Check sheet for the modelled part. Datum: model origin and axes. Units: mm. A direction names the side the tool comes from. Round coordinates to 2 decimals unless told otherwise and drop trailing zeros. Loops run counter-clockwise (first coordinate to the right, second up) from the corner with the lowest first, then second, coordinate; pieces in that order, holes last. Notation, with made-up numbers: (30, 9) - (42, 9) arc R10 ccw to (42, 22) - close; hole circle Ø10 at (49.25, -6.5). An arc over 180 degrees is marked (long way). Put each result on its own line as item: value. Start each with the question number.
Item 1: Tool access check on faces 4 (the flat face through (-7, 0, 0)), 5 (the flat face through (-6.096, 13, 0)). Record the directions out of +Z, -Z, +X, -X, +Y, -Y that give a thin tool (end or side, any length) a straight path to the whole face; none if there is none.
Item 2: Draft check along X on faces 1 (the flat face through (0, 13, 8)), 2 (the flat face through (-4, 13, 12)), 3 (the flat face through (-3.09, 12.52, 6.3)). Enter one of: pulls with the +X half, pulls with the -X half, needs draft (parallel to the pull), parting line crosses it, or undercut.
Item 3: Section check C-C, the plane x = -2.5. Record the cut outline in (y, z), and give its area (3 significant figures).
Item 4: Section check B-B, the plane y = 14.5. Record the cut outline in (x, z).
Item 5: Section check A-A, the plane x = -1.25. Record the cut outline in (y, z).
Item 6: Section check D-D, the plane z = 0. Record the cut outline in (x, y).
Item 7: Material ranges on line 1 along X through (y, z) = (7, -4.5); line 2 along Z through (x, y) = (-0.75, 14); line 3 along Z through (x, y) = (-5.25, 20.5), recorded low to high.
Autodesk Inventor part; units mm, degrees
ref_plane "YZ Plane" through (0, 0, 0) normal (1, 0, 0) x (0, 1, 0)
ref_plane "XZ Plane" through (0, 0, 0) normal (0, 1, 0) x (-1, 0, 0)
ref_plane "XY Plane" through (0, 0, 0) normal (0, 0, 1) x (1, 0, 0)
sketch "Sketch1" plane through (0, 0, 0) normal (0, 1, 0) x (-1, 0, 0)
  line L0 (0, 12) -> (7.366, 12)
  line L1 (7.366, 12) -> (7.366, -12)
  line L2 (7.366, -12) -> (0, -12)
  line L3 (6.096, 4.754) -> (6.096, -4.754)
  line L4 (0, 4.754) -> (0, 7.802)
  line L5 (6.096, 7.802) -> (6.096, 4.754)
  line L6 (0, -4.754) -> (0, -7.548)
  line L7 (6.096, -7.802) -> (6.096, -4.754)
  line L8 (6.096, 7.802) -> (0, 4.754)
  line L9 (6.096, -7.802) -> (0, -4.754)
  line L10 (0, -12) -> (0, -4.754)
  line L11 (0, 4.754) -> (0, 12)
  point P0 (0, 0)
  dimension "d0" = 7.366
  dimension "d1" = 24
  dimension "d2" = 12
  dimension "d8" = 9.508
  dimension "d9" = 4.754
  dimension "d10" = 3.048
  dimension "d11" = 3.048
  dimension "d12" = 6.096
extrude "Extrusion1" add sketch "Sketch1" along normal blind 25.4
equation "\"d11\" = d10"
properties part number "Sliding test receiver"
Check result:
1. face 4: +Z, -Z, +X, -X, -Y
1. face 5: +Y, -Y
2. face 1: pulls with the +X half
2. face 2: needs draft
2. face 3: undercut
3. outline: (0, -12) - (25.4, -12) - (25.4, -6) - (0, -6) - close; (0, 6) - (25.4, 6) - (25.4, 12) - (0, 12) - close
3. area: 305 mm²
4. outline: (-7.37, -12) - (0, -12) - (0, -4.75) - (-6.1, -7.8) - (-6.1, 7.8) - (0, 4.75) - (0, 12) - (-7.37, 12) - close
5. outline: (0, -12) - (25.4, -12) - (25.4, -5.38) - (0, -5.38) - close; (0, 5.38) - (25.4, 5.38) - (25.4, 12) - (0, 12) - close
6. outline: (-7.37, 0) - (-6.1, 0) - (-6.1, 25.4) - (-7.37, 25.4) - close
7. line 1: -7.37 to -6.1
7. line 2: -12 to -5.13, 5.13 to 12
7. line 3: -12 to -7.38, 7.38 to 12
